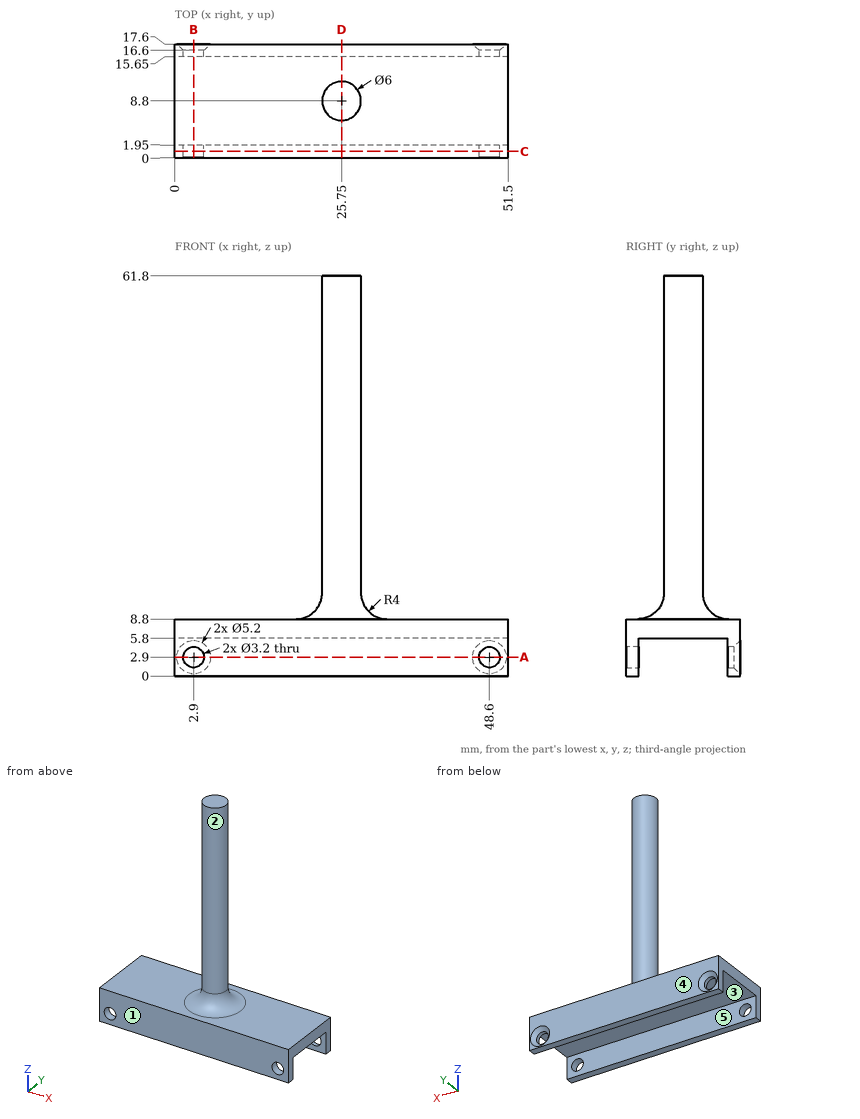
Check sheet for the drawn part. Datum: minimum x, y, z corner. Units: mm. A direction names the side the tool comes from. Give positions to 0.01 mm unless a question says otherwise; leave off trailing zeros. Order: outer loops, then holes, each group sorted by start corner. A loop starts at its lowest first (then second) coordinate and runs counter-clockwise, first axis right, second up. Notation, with made-up numbers: (-14.5, -39.75) -> (8.5, -39.75) arc R35 cw to (8.5, -0.75) -> close; hole circle Ø4 at (-12, 38). An arc over 180 degrees is marked (long way). Use a Markdown table: item, result.
1) Mould release check, pull along Y, two halves, no side actions. Record for the marked faces 1, 2 and 3: pulls with the +Y half, pulls with the -Y half, needs draft (parallel to the pull), parting line crosses it, or undercut.
Results:
| item | result |
|---|---|
| face 1 | pulls with the -Y half |
| face 2 | parting line crosses it |
| face 3 | undercut |
2) Section check B-B, the plane x = 2.9. Record the boundary of the cut face in (y, z).
Results:
| item | result |
|---|---|
| outline | (0, 0) -> (1.95, 0) -> (1.95, 1.3) -> (0, 1.3) -> close; (0, 4.5) -> (1.95, 4.5) -> (1.95, 5.8) -> (15.65, 5.8) -> (15.65, 4.5) -> (16.6, 4.5) -> (17.6, 5.5) -> (17.6, 8.8) -> (0, 8.8) -> close; (15.65, 0) -> (17.6, 0) -> (17.6, 0.3) -> (16.6, 1.3) -> (15.65, 1.3) -> close |
3) Section check C-C, the plane y = 1. Record the boundary of the cut face in (x, z), then the cut area to 3 significant figures.
Results:
| item | result |
|---|---|
| outline | (0, 0) -> (51.5, 0) -> (51.5, 8.8) -> (0, 8.8) -> close; hole circle Ø3.2 at (2.9, 2.9); hole circle Ø3.2 at (48.6, 2.9) |
| area | 437 mm² |
4) Section check A-A, the plane z = 2.9. Record the boundary of the cut face in (x, y).
Results:
| item | result |
|---|---|
| outline | (0, 0) -> (1.3, 0) -> (1.3, 1.95) -> (0, 1.95) -> close; (0, 15.65) -> (1.3, 15.65) -> (1.3, 16.6) -> (0.3, 17.6) -> (0, 17.6) -> close; (4.5, 0) -> (47, 0) -> (47, 1.95) -> (4.5, 1.95) -> close; (4.5, 15.65) -> (47, 15.65) -> (47, 16.6) -> (46, 17.6) -> (5.5, 17.6) -> (4.5, 16.6) -> close; (50.2, 0) -> (51.5, 0) -> (51.5, 1.95) -> (50.2, 1.95) -> close; (50.2, 15.65) -> (51.5, 15.65) -> (51.5, 17.6) -> (51.2, 17.6) -> (50.2, 16.6) -> close |
5) Depth check by flat-ended pin: pin 1 Ø10 at (y, z) = (6.5, 20.5) entering from +X; pin 2 Ø9 at (x, y) = (17.5, 8) entering from +Z; pin 3 Ø4 at (x, z) = (48.6, 2.9) entering from +Y. Enter the tip coordinate at first touch or a pass-through.
Results:
| item | result |
|---|---|
| pin 1 | x = 28.75 |
| pin 2 | z = 10.42 |
| pin 3 | y = 17 |
6) Section check D-D, the plane x = 25.75. Record the boundary of the cut face in (y, z), then the cut area to 3 significant figures.
Results:
| item | result |
|---|---|
| outline | (0, 0) -> (1.95, 0) -> (1.95, 5.8) -> (15.65, 5.8) -> (15.65, 0) -> (17.6, 0) -> (17.6, 8.8) -> (15.8, 8.8) arc R4 cw to (11.8, 12.8) -> (11.8, 61.8) -> (5.8, 61.8) -> (5.8, 12.8) arc R4 cw to (1.8, 8.8) -> (0, 8.8) -> close |
| area | 400 mm² |
7) Tool access check on the marked faces 4 and 5. Record the directions out of +Z, -Z, +X, -X, +Y, -Y that give a thin tool (end or side, any length) a straight path to the whole face; none if there is none.
Results:
| item | result |
|---|---|
| face 4 | +Z, -Z, +X, -X, +Y |
| face 5 | -Z, +X, -X |
8) Material ranges on probe 1 along X at (y, z) = (15.9, 2.9); probe 2 along Z at (x, y) = (47.5, 10.75); probe 3 along Z at (x, y) = (27.5, 9), recorded low to high.
Results:
| item | result |
|---|---|
| probe 1 | 0 to 1.3, 4.5 to 47, 50.2 to 51.5 |
| probe 2 | 5.8 to 8.8 |
| probe 3 | 5.8 to 61.8 |
